```python
from build123d import *

# Parameters (mm, degrees)
SKETCH1_W           = 50.8
SKETCH1_H           = 3.175
BOSS_EXTRUDE1_DEPTH = 69.85
SKETCH2_W           = 6.35
SKETCH2_H           = 6.35
SKETCH2_W_2         = 12.7
CUT_EXTRUDE1_DEPTH  = 325.41579514


with BuildPart() as part:
    # Sketch1 → Boss-Extrude1 (new body)
    with BuildSketch(Plane.XY):
        with Locations((291.390948437, 357.142928402)):
            Rectangle(SKETCH1_W, SKETCH1_H)
    extrude(amount=-BOSS_EXTRUDE1_DEPTH)

    # Sketch2 → Cut-Extrude1 (cut, through all)
    with BuildSketch(Plane(origin=(0, 358.730428402, 0), x_dir=(1, 0, 0), z_dir=(0, 1, 0))):
        with Locations((269.165948437, 66.675)):
            Rectangle(SKETCH2_W, SKETCH2_H)
        with Locations((313.615948437, 66.675)):
            Rectangle(SKETCH2_W, SKETCH2_H)
        with Locations((291.390948437, 66.675)):
            Rectangle(SKETCH2_W_2, SKETCH2_H)
        with Locations((269.165948437, 3.175)):
            Rectangle(SKETCH2_W, SKETCH2_H)
        with Locations((291.390948437, 3.175)):
            Rectangle(SKETCH2_W_2, SKETCH2_H)
        with Locations((313.615948437, 3.175)):
            Rectangle(SKETCH2_W, SKETCH2_H)
    extrude(amount=-CUT_EXTRUDE1_DEPTH, mode=Mode.SUBTRACT)


solid = part.part
```
For this review, take the finished solid that the model builds, in its own axes (mm). A direction names the side the tool comes from. Round coordinates to 2 decimals unless told otherwise and drop trailing zeros. Write each loop counter-clockwise with the first axis right and the second up, starting at its lowest first coordinate (ties: lowest second). Pieces come first, ordered by that corner, then holes. Notation, with made-up numbers: M 59,9.25 L 105,9.25 A15 ccw 105,33.25 Z; hole C 76,-13 d6. An arc over 180 degrees is marked long. One line per item, written item: value. Start each with the question number.
(1) Insertion check: pin 1 (1.5 mm diameter, centred on x = 297.5, y = 358, fed in from +Z); pin 2 (1 mm diameter, centred on x = 290, y = 356.5, fed in from +Z); pin 3 (1.6 mm diameter, centred on y = 358, z = -66, fed in from -X); pin 4 (1 mm diameter, centred on y = 357.5, z = -66, fed in from +X). Each pin has a flat end and moves straight along its axis. Give the tip position at first contact, or say it passes through.
(2) The part is to be moulded in two halves that separate along X. For faces 1 (the flat face through (285.041, 357, -3)), 2 (the flat face through (265.991, 357, -35)), 3 (the flat face through (279, 357, 0)), say which applies: released by +X, released by -X, zero draft, split by the parting line, or undercut.
(3) Wall thickness on line 1 (X direction, y = 357.85, z = -66.5); line 2 (Z direction, x = 290, y = 357.05): over which ranges is each line inside the solid? List them lowest first.
(4) Machinability: for faces 4 (the flat face through (269, 357, -6.35)), 5 (the flat face through (297.741, 357, -67)), 6 (the flat face through (310.441, 357, -67)), which of the approach directions +Z, -Z, +X, -X, +Y, -Y give a long, thin tool a straight path to every point of the face, cutting with its end or side? Answer none if there is none.
(5) We need section A-A (y = 357.85). Give the boundary of the cut face in (x, z), and give its area (3 significant figures).
(6) We need section B-B (x = 312.5). Give the boundary of the cut face in (y, z).
Result:
1. pin 1: z = 0
1. pin 2: z = -6.35
1. pin 3: x = 272.34
1. pin 4: x = 310.44
2. face 1: undercut
2. face 2: released by -X
2. face 3: zero draft
3. line 1: 272.34 to 285.04, 297.74 to 310.44
3. line 2: -63.5 to -6.35
4. face 4: +Z, -X, +Y, -Y
4. face 5: -Z, +Y, -Y
4. face 6: -Z, +X, +Y, -Y
5. outline: M 265.99,-63.5 L 272.34,-63.5 L 272.34,-69.85 L 285.04,-69.85 L 285.04,-63.5 L 297.74,-63.5 L 297.74,-69.85 L 310.44,-69.85 L 310.44,-63.5 L 316.79,-63.5 L 316.79,-6.35 L 310.44,-6.35 L 310.44,0 L 297.74,0 L 297.74,-6.35 L 285.04,-6.35 L 285.04,0 L 272.34,0 L 272.34,-6.35 L 265.99,-6.35 Z
5. area: 3,230 mm²
6. outline: M 355.56,-63.5 L 358.73,-63.5 L 358.73,-6.35 L 355.56,-6.35 Z
